Design review of the part built by this model. Coordinates are the model's own, in mm. A direction names the side the tool comes from. Round coordinates to 2 decimals unless told otherwise and drop trailing zeros. Write each loop counter-clockwise with the first axis right and the second up, starting at its lowest first coordinate (ties: lowest second). Pieces come first, ordered by that corner, then holes. Notation, with made-up numbers: M -8.75,60 L 18.25,60 A29 ccw 18.25,94 Z; hole C 63.25,56.25 d7. An arc over 180 degrees is marked long. Use CSV: the item, a comma, the result in double quotes.
Autodesk Inventor part; units mm, degrees
ref_plane "YZ Plane" through (0, 0, 0) normal (1, 0, 0) x (0, 1, 0)
ref_plane "XZ Plane" through (0, 0, 0) normal (0, 1, 0) x (-1, 0, 0)
ref_plane "XY Plane" through (0, 0, 0) normal (0, 0, 1) x (1, 0, 0)
sketch "Sketch1" plane through (0, 0, 0) normal (0, 1, 0) x (-1, 0, 0)
  line L0 (0, 0) -> (57, 0)
  line L1 (57, 0) -> (57, 5)
  line L2 (57, 5) -> (0, 5)
  line L3 (0, 5) -> (0, 0)
  circle A0 centre (54.5, 2.5) radius 2.5
  circle A1 centre (2.5, 2.5) radius 2.5
  circle A2 centre (54.5, 2.5) radius 5
  circle A3 centre (2.5, 2.5) radius 5
  line L4 (57, 0) -> (57, 5)
  line L5 (57, 2.5) -> (0, 2.5)
  point P0 (50.1699, 0)
  point P1 (50.1699, 5)
  point P2 (6.8301, 5)
  point P3 (6.8301, 0)
  dimension "d0" = 5
  dimension "d1" = 57
  dimension "d2" = 5
  dimension "d3" = 5
  dimension "d4" = 10
  dimension "d5" = 10
extrude "Extrusion1" add sketch "Sketch1" along normal blind 2.7 contours L3 A1 L0 | L0 A3 L2 L3 | A1 L5 A3 L0 | L3 L2 A1 | A3 L5 A2 L0 | A1 L2 A3 L5 | A2 L5 A0 L0 | L0 L1 L2 A2 | L2 A2 L5 A3 | A0 L1 L0 | A2 L2 A0 L5 | A0 L2 L1
properties part number "FP V2 Batang Penggerak" material "Aluminum 6061"
1) Wall thickness on line 1 along X through (y, z) = (1, 2.5); line 2 along Z through (x, y) = (-54.5, 1); line 3 along X through (y, z) = (2.5, 0.75): over which ranges is each line inside the solid? List them lowest first. Write a range as [from, to].
Answers:
line 1,"[-59.5, -57], [-52, -5], [0, 2.5]"
line 2,"[-2.5, 0], [5, 7.5]"
line 3,"[-59.18, -56.29], [-52.71, -4.29], [-0.71, 2.18]"
2) Add section C-C on y = 0.55. Write out the cut boundary in (x, z), then the cut area to 3 significant figures.
Answers:
outline,"M -50.17,0 L -6.83,0 A5 ccw long -6.83,5 L -50.17,5 A5 ccw long Z; hole C -54.5,2.5 d5; hole C -2.5,2.5 d5"
area,"330 mm²"
3) Add section B-B on z = 2.5. Write out the cut boundary in (x, y), then the cut area to 3 significant figures.
Answers:
outline,"M -59.5,0 L -57,0 L -57,2.7 L -59.5,2.7 Z; M -52,0 L -5,0 L -5,2.7 L -52,2.7 Z; M 0,0 L 2.5,0 L 2.5,2.7 L 0,2.7 Z"
area,"140 mm²"
4) Machinability: for faces 5 (the face through (-29, 1, 5)), 6 (the face through (-28, 2.7, 3)), 7 (the face through (-28, 1, 0)), which of the approach directions +Z, -Z, +X, -X, +Y, -Y give a long, thin tool a straight path to every point of the face, cutting with its end or side? Answer none if there is none.
Answers:
face 5,"+Z, +Y, -Y"
face 6,"+Z, -Z, +X, -X, +Y"
face 7,"-Z, +Y, -Y"
5) Add section D-D on x = -31.5. Write out the cut boundary in (y, z).
Answers:
outline,"M 0,0 L 2.7,0 L 2.7,5 L 0,5 Z"
6) The part is to be moulded in two halves that separate along Z. For faces 1 (the face through (-28, 0, 3)), 2 (the face through (-0.5, 1.3, 4)), 3 (the face through (-56.81, 1.33, 3.46)), 4 (the face through (2.497, 1.331, 2.317)), say which applies: released by +Z, released by -Z, zero draft, split by the parting line, or undercut.
Answers:
face 1,"zero draft"
face 2,"undercut"
face 3,"undercut"
face 4,"split by the parting line"
7) For pin 1 Ø1 at (x, y) = (-22.5, 1.5) entering from +Z; pin 2 Ø1.5 at (y, z) = (2, 4.5) entering from -X, all flat-tipped, find the tip position at first contact; note any pin that passes through.
Answers:
pin 1,"z = 5"
pin 2,"x = -59.34"
8) Add section A-A on x = -54.5. Write out the cut boundary in (y, z).
Answers:
outline,"M 0,-2.5 L 2.7,-2.5 L 2.7,0 L 0,0 Z; M 0,5 L 2.7,5 L 2.7,7.5 L 0,7.5 Z"
